Geometry check sheet. Reference: the model listing, model coordinates, mm. Give positions to 0.01 mm unless a question says otherwise; leave off trailing zeros. Write each loop counter-clockwise with the first axis right and the second up, starting at its lowest first coordinate (ties: lowest second). Pieces come first, ordered by that corner, then holes.
(1) Cross-section at A-A (x = 0). Record the boundary of the cut face in (y, z), and give its area (3 significant figures).
(2) Cross-section at B-B (z = 0). Record the boundary of the cut face in (x, y).
(3) Cross-section at C-C (y = 1.95). Count the separate pieces of the cut face and the enclosed holes in it, and give its area (3 significant figures).
(4) Thickness scan on line 1 along Z through (x, y) = (-0.5, 3); line 2 along X through (y, z) = (3.3, 56); line 3 along X through (y, z) = (0.95, 65.5). Record the ranges inside material, lowest first.
(5) Depth check by flat-ended pin: P1, Ø2.5, axis at y = 1.5, z = -31, coming from the +X side; P2, Ø1, axis at x = 40.5, y = 1.5, coming from the +Z side; P3, Ø1.5, axis at y = 3, z = 39, coming from the +X side; P4, Ø16, axis at x = 37.5, z = -64.95, coming from the -Y side. Enter the tip coordinate at first touch or a pass-through.
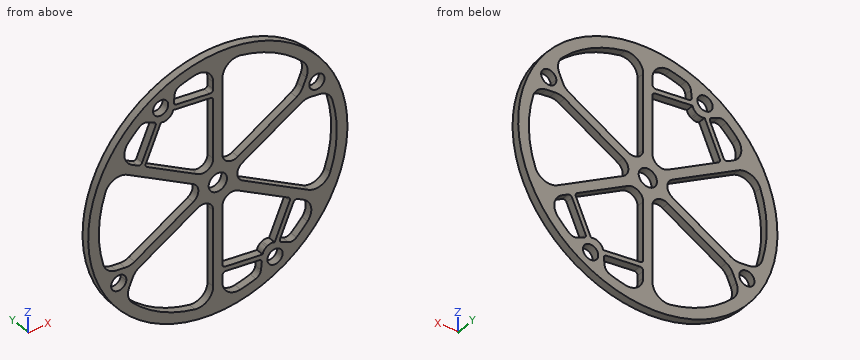
```python
from build123d import *

# Parameters (mm, degrees)
SZKIC1_R                    = 85
DODANIE_WYCI_GNI_CIE1_DEPTH = 5
SZKIC2_R                    = 5
SZKIC2_R_2                  = 6
WYTNIJ_WYCI_GNI_CIE2_DEPTH  = 5
ZAOKR_GLENIE2_R             = 10
ZAOKR_GLENIE4_R             = 10
ZAOKR_GLENIE5_R             = 5
DODANIE_WYCI_GNI_CIE2_DEPTH = 5
ZAOKR_GLENIE6_R             = 2


with BuildPart() as part:
    # Szkic1 → Dodanie-wyciągnięcie1 (new body)
    with BuildSketch(Plane(origin=(0, 0, 0), x_dir=(1, 0, 0), z_dir=(0, 1, 0))):
        with Locations(Location((0, 0, 0), (0, 0, 270))):
            Circle(SZKIC1_R)
    extrude(amount=DODANIE_WYCI_GNI_CIE1_DEPTH)

    # Szkic2 → Wytnij-wyciągnięcie2 (cut)
    with BuildSketch(Plane(origin=(0, 5, 0), x_dir=(1, 0, 0), z_dir=(0, 1, 0))):
        with BuildLine():
            Line((3, 77.942286341), (3, 16.907164233))
            ThreePointArc((3, 16.907164233), (6.38067791, 11.051658328), (13.142033731, 11.051658328))
            Line((13.142033731, 11.051658328), (66, 41.569219382))
            ThreePointArc((66, 41.569219382), (58.334842927, 51.778819035), (49.106893514, 60.601262441))
            Line((49.106893514, 60.601262441), (34.87960923, 54.413255334))
            ThreePointArc((34.87960923, 54.413255334), (32.316363874, 55.973584145), (29.683456807, 57.413255334))
            Line((29.683456807, 57.413255334), (27.928786019, 72.828448504))
            ThreePointArc((27.928786019, 72.828448504), (15.674351199, 76.408865418), (3, 77.942286341))
        make_face()
        with BuildLine():
            ThreePointArc((-13.142033731, 11.051658328), (-6.38067791, 11.051658328), (-3, 16.907164233))
            Line((-3, 16.907164233), (-3, 77.942286341))
            ThreePointArc((-3, 77.942286341), (-34.916330218, 69.748475855), (-60.601262441, 49.106893514))
            Line((-60.601262441, 49.106893514), (-54.413255334, 34.87960923))
            Line((-54.413255334, 34.87960923), (-13.142033731, 11.051658328))
        make_face()
        with BuildLine():
            Line((69, 36.373066959), (16.142033731, 5.855505905))
            ThreePointArc((16.142033731, 5.855505905), (12.761355821, 0), (16.142033731, -5.855505905))
            Line((16.142033731, -5.855505905), (57.413255334, -29.683456807))
            Line((57.413255334, -29.683456807), (72.828448504, -27.928786019))
            ThreePointArc((72.828448504, -27.928786019), (77.862117075, 4.635808952), (69, 36.373066959))
        make_face()
        with BuildLine():
            ThreePointArc((-16.142033731, -5.855505905), (-12.761355821, 0), (-16.142033731, 5.855505905))
            Line((-16.142033731, 5.855505905), (-57.413255334, 29.683456807))
            Line((-57.413255334, 29.683456807), (-72.828448504, 27.928786019))
            ThreePointArc((-72.828448504, 27.928786019), (-77.862117075, -4.635808952), (-69, -36.373066959))
            Line((-69, -36.373066959), (-16.142033731, -5.855505905))
        make_face()
        with BuildLine():
            ThreePointArc((-62.987803669, 32.901923789), (-60.621778265, 35), (-59.987803669, 38.098076211))
            ThreePointArc((-59.987803669, 38.098076211), (-69.282032303, 40), (-62.987803669, 32.901923789))
        make_face()
        with BuildLine():
            ThreePointArc((59.987803669, -38.098076211), (69.282032303, -40), (62.987803669, -32.901923789))
            ThreePointArc((62.987803669, -32.901923789), (60.621778265, -35), (59.987803669, -38.098076211))
        make_face()
        with BuildLine():
            Line((60.601262441, -49.106893514), (54.413255334, -34.87960923))
            Line((54.413255334, -34.87960923), (13.142033731, -11.051658328))
            ThreePointArc((13.142033731, -11.051658328), (6.38067791, -11.051658328), (3, -16.907164233))
            Line((3, -16.907164233), (3, -77.942286341))
            ThreePointArc((3, -77.942286341), (34.916330218, -69.748475855), (60.601262441, -49.106893514))
        make_face()
        with BuildLine():
            ThreePointArc((-3, -16.907164233), (-6.38067791, -11.051658328), (-13.142033731, -11.051658328))
            Line((-13.142033731, -11.051658328), (-66, -41.569219382))
            ThreePointArc((-66, -41.569219382), (-58.334842927, -51.778819035), (-49.106893514, -60.601262441))
            Line((-49.106893514, -60.601262441), (-34.87960923, -54.413255334))
            ThreePointArc((-34.87960923, -54.413255334), (-32.316363874, -55.973584145), (-29.683456807, -57.413255334))
            Line((-29.683456807, -57.413255334), (-27.928786019, -72.828448504))
            ThreePointArc((-27.928786019, -72.828448504), (-15.674351199, -76.408865418), (-3, -77.942286341))
            Line((-3, -77.942286341), (-3, -16.907164233))
        make_face()
        with Locations(Location((-37.5, -64.951905284, 0), (0, 0, 270))):
            Circle(SZKIC2_R)
        with Locations(Location((37.5, 64.951905284, 0), (0, 0, 270))):
            Circle(SZKIC2_R)
        with Locations(Location((0, 0, 0), (0, 0, 270))):
            Circle(SZKIC2_R_2)
    extrude(amount=-WYTNIJ_WYCI_GNI_CIE2_DEPTH, mode=Mode.SUBTRACT)

    # Zaokrąglenie2
    zaokr_glenie2_edges = [part.edges().sort_by_distance(p)[0] for p in [
        (-60.601262441, 2.5, -49.106893514),
        (-3, 2.5, -77.942286341),
        (-69, 2.5, 36.373066959),
        (-72.828448504, 2.5, -27.928786019),
        (69, 2.5, -36.373066959),
        (72.828448504, 2.5, 27.928786019),
        (3, 2.5, -77.942286341),
        (66, 2.5, -41.569219382),
        (60.601262441, 2.5, 49.106893514),
        (3, 2.5, 77.942286341),
        (-3, 2.5, 77.942286341),
        (-66, 2.5, 41.569219382),
    ]]
    fillet(zaokr_glenie2_edges, radius=ZAOKR_GLENIE2_R)

    # Zaokrąglenie4
    zaokr_glenie4_edges = [part.edges().sort_by_distance(p)[0] for p in [
        (-54.413255334, 2.5, -34.87960923),
        (-57.413255334, 2.5, -29.683456807),
        (57.413255334, 2.5, 29.683456807),
        (54.413255334, 2.5, 34.87960923),
    ]]
    fillet(zaokr_glenie4_edges, radius=ZAOKR_GLENIE4_R)

    # Zaokrąglenie5
    zaokr_glenie5_edges = [part.edges().sort_by_distance(p)[0] for p in [
        (27.928786019, 2.5, -72.828448504),
        (29.683456807, 2.5, -57.413255334),
        (34.87960923, 2.5, -54.413255334),
        (49.106893514, 2.5, -60.601262441),
        (-27.928786019, 2.5, 72.828448504),
        (-29.683456807, 2.5, 57.413255334),
        (-34.87960923, 2.5, 54.413255334),
        (-49.106893514, 2.5, 60.601262441),
    ]]
    fillet(zaokr_glenie5_edges, radius=ZAOKR_GLENIE5_R)

    # Szkic3 → Dodanie-wyciągnięcie2 (add, through all)
    with BuildSketch(Plane(origin=(0, 5, 0), x_dir=(1, 0, 0), z_dir=(0, 1, 0))):
        Polygon((3, 57), (29.388588378, 60.003743428), (29.049297257, 62.984495269), (3, 60.019372454), align=None)
        Polygon((40.021524319, 56.649677021), (37.270471942, 55.453135831), (47.863448016, 31.098076211), (50.478301265, 32.607762438), align=None)
        Polygon((-47.863448016, -31.098076211), (-37.270471942, -55.453135831), (-40.021524319, -56.649677021), (-50.478301265, -32.607762438), align=None)
        Polygon((-3, -60.019372454), (-3, -57), (-29.388588378, -60.003743428), (-29.049297257, -62.984495269), align=None)
    extrude(amount=-DODANIE_WYCI_GNI_CIE2_DEPTH)

    # Zaokrąglenie6
    zaokr_glenie6_edges = [part.edges().sort_by_distance(p)[0] for p in [
        (3, 2.5, -57),
        (3, 2.5, -60.019372454),
        (29.049297257, 2.5, -62.984495269),
        (40.021524319, 2.5, -56.649677021),
        (50.478301265, 2.5, -32.607762438),
        (47.863448016, 2.5, -31.098076211),
        (-50.478301265, 2.5, 32.607762438),
        (-47.863448016, 2.5, 31.098076211),
        (-40.021524319, 2.5, 56.649677021),
        (-3, 2.5, 60.019372454),
        (-29.049297257, 2.5, 62.984495269),
        (-3, 2.5, 57),
    ]]
    fillet(zaokr_glenie6_edges, radius=ZAOKR_GLENIE6_R)


solid = part.part
```
Reply:
1. outline: (0, -85) - (5, -85) - (5, -6) - (0, -6) - close; (0, 6) - (5, 6) - (5, 85) - (0, 85) - close
1. area: 790 mm2
2. outline: (-85, 0) - (-78, 0) - (-78, 5) - (-85, 5) - close; (-12.76, 0) - (-6, 0) - (-6, 5) - (-12.76, 5) - close; (6, 0) - (12.76, 0) - (12.76, 5) - (6, 5) - close; (78, 0) - (85, 0) - (85, 5) - (78, 5) - close
3. separate pieces: 1
3. enclosed holes: 15
3. area: 7,320 mm2
4. line 1: z = -85 to -5.98, 5.98 to 85
4. line 2: x = -63.95 to -54.3, -40.69 to -32.27, -3.16 to 3, 54.3 to 63.95
4. line 3: x = -54.17 to -42.47, -32.53 to -28.76, -3 to 3, 42.35 to 54.17
5. P1: stops at x = 79.62
5. P2: stops at z = 75
5. P3: stops at x = 75.91
5. P4: stops at y = 0
